Model file for the job. Use its own axes, mm. Coordinates: 2 decimals unless noted, no trailing zeros. Order: outer loops, then holes, each group sorted by start corner. A loop starts at its lowest first (then second) coordinate and runs counter-clockwise, first axis right, second up.
from build123d import *

# Parameters (mm, degrees)
SKETCH1_W           = 30.16
SKETCH1_H           = 39.56
SKETCH1_R           = 1.5875
SKETCH1_W_2         = 4.521190227
SKETCH1_H_2         = 4.521190227
SKETCH1_W_3         = 4.521190228
SKETCH1_H_3         = 4.521190228
BOSS_EXTRUDE1_DEPTH = 5.588
CHAMFER1_SIZE       = 10
CHAMFER2_SIZE       = 4


with BuildPart() as part:
    # Sketch1 → Boss-Extrude1 (new body)
    with BuildSketch(Plane(origin=(0, 0, 0), x_dir=(0, 0, -1), z_dir=(1, 0, 0))):
        with Locations((4.886e-06, 4.886e-06)):
            Rectangle(SKETCH1_W, SKETCH1_H)
        with Locations((-10.079995114, 12.700004886)):
            Circle(SKETCH1_R, mode=Mode.SUBTRACT)
        with Locations((-10.079995114, -12.699995114)):
            Circle(SKETCH1_R, mode=Mode.SUBTRACT)
        with Locations((10.080004886, 0)):
            Circle(SKETCH1_R, mode=Mode.SUBTRACT)
        with Locations((4.886e-06, 12.700004887)):
            Rectangle(SKETCH1_W_2, SKETCH1_H_2, mode=Mode.SUBTRACT)
        Rectangle(SKETCH1_W_3, SKETCH1_H_3, mode=Mode.SUBTRACT)
        with Locations((4.886e-06, -12.699995114)):
            Rectangle(SKETCH1_W_2, SKETCH1_H_2, mode=Mode.SUBTRACT)
    extrude(amount=BOSS_EXTRUDE1_DEPTH)

    # Chamfer1
    chamfer1_edges = [part.edges().sort_by_distance(p)[0] for p in [
        (2.794, 19.780004886, -15.080004886),
        (2.794, -19.779995114, -15.080004886),
    ]]
    chamfer(chamfer1_edges, length=CHAMFER1_SIZE)

    # Chamfer2
    chamfer2_edges = [part.edges().sort_by_distance(p)[0] for p in [
        (2.794, 19.780004886, 15.079995114),
        (2.794, -19.779995114, 15.079995114),
    ]]
    chamfer(chamfer2_edges, length=CHAMFER2_SIZE)


solid = part.part
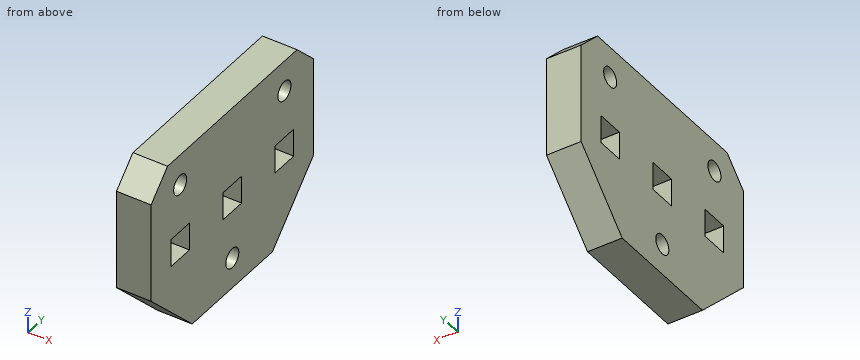
Q1. Cut at B-B, the plane z = 1. List the corners of the cut face in (x, y), plus the area to 3 significant figures.
Established:
outline: (0, -19.78) - (5.59, -19.78) - (5.59, -14.96) - (0, -14.96) - close; (0, -10.44) - (5.59, -10.44) - (5.59, -2.26) - (0, -2.26) - close; (0, 2.26) - (5.59, 2.26) - (5.59, 10.44) - (0, 10.44) - close; (0, 14.96) - (5.59, 14.96) - (5.59, 19.78) - (0, 19.78) - close
area: 145 mm2
Q2. Probe line 1 (Y direction, x = 0.7, z = 10); line 2 (Y direction, x = 0.3, z = 0); line 3 (Z direction, x = 0.8, y = -12.5). List the from-to ranges inside material, lowest first.
Established:
line 1: y = -19.78 to -14.29, -11.11 to 11.11, 14.29 to 19.78
line 2: y = -19.78 to -14.96, -10.44 to -2.26, 2.26 to 10.44, 14.96 to 19.78
line 3: z = -12.36 to -2.26, 2.26 to 8.51, 11.65 to 15.08
Q3. Drop flat-ended pins along their axis: P1, Ø1.4, axis at x = 3.5, y = 12, coming from the -Z side; P2, Ø3, axis at y = 12.7, z = 10.08, coming from the +X side; P3, Ø3, axis at x = 0.5, y = -14, coming from the -Z side. Give the stop position or say it passes through.
Established:
P1: stops at z = -13.56
P2: passes through
P3: stops at z = -12.36
Q4. Cut at A-A, the plane y = 0. List the corners of the cut face in (x, z).
Established:
outline: (0, -15.08) - (5.59, -15.08) - (5.59, -11.67) - (0, -11.67) - close; (0, -8.49) - (5.59, -8.49) - (5.59, -2.26) - (0, -2.26) - close; (0, 2.26) - (5.59, 2.26) - (5.59, 15.08) - (0, 15.08) - close
Q5. Cut at C-C, the plane x = 2.2. List the corners of the cut face in (y, z) (1 decimal), plus the area to 3 significant figures.
Established:
outline: (-19.8, -5.1) - (-9.8, -15.1) - (9.8, -15.1) - (19.8, -5.1) - (19.8, 11.1) - (15.8, 15.1) - (-15.8, 15.1) - (-19.8, 11.1) - close; hole (-15, -2.3) - (-10.4, -2.3) - (-10.4, 2.3) - (-15, 2.3) - close; hole circle Ø3.2 at (-12.7, 10.1); hole (-2.3, -2.3) - (2.3, -2.3) - (2.3, 2.3) - (-2.3, 2.3) - close; hole circle Ø3.2 at (0, -10.1); hole (10.4, -2.3) - (15, -2.3) - (15, 2.3) - (10.4, 2.3) - close; hole circle Ø3.2 at (12.7, 10.1)
area: 992 mm2
Q6. Cut at D-D, the plane z = -9.5. List the corners of the cut face in (x, y), plus the area to 3 significant figures.
Established:
outline: (0, -15.36) - (5.59, -15.36) - (5.59, -1.48) - (0, -1.48) - close; (0, 1.48) - (5.59, 1.48) - (5.59, 15.36) - (0, 15.36) - close
area: 155 mm2
